Build history of the part. All positions in model axes, mm. Face numbers are marked on the shaded views. Round coordinates to 2 decimals unless told otherwise and drop trailing zeros. Loops run counter-clockwise (first coordinate to the right, second up) from the corner with the lowest first, then second, coordinate; pieces in that order, holes last. Notation, with made-up numbers: (74, -26.5) - (119, -26.5) arc R35 ccw to (119, 11.5) - close; hole circle Ø9 at (4.5, -9.5). An arc over 180 degrees is marked (long way). Use a Markdown table: item, result.
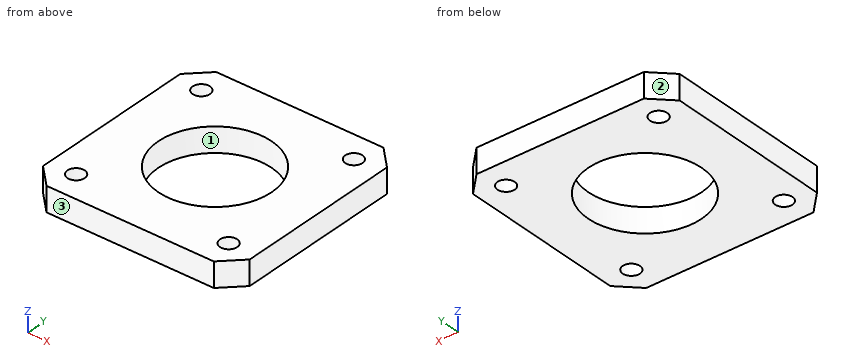
from build123d import *

# Parameters (mm, degrees)
SKETCH_W        = 42
SKETCH_H        = 42
PAD_DEPTH       = 5
SKETCH001_R     = 11.5
POCKET_DEPTH    = 12
SKETCH002_R     = 1.75
POCKET001_DEPTH = 12
CHAMFER_SIZE    = 4


with BuildPart() as part:
    # Sketch → Pad (new body)
    with BuildSketch(Plane.XY):
        Rectangle(SKETCH_W, SKETCH_H)
    extrude(amount=PAD_DEPTH)

    # Sketch001 (on Face6 of Pad) → Pocket (cut)
    with BuildSketch(Plane.XY.offset(5)):
        Circle(SKETCH001_R)
    extrude(amount=-POCKET_DEPTH, mode=Mode.SUBTRACT)

    # Sketch002 (on Face5 of Pocket) → Pocket001 (cut)
    with BuildSketch(Plane.XY.offset(5)):
        with Locations((15.5, 15.5)):
            Circle(SKETCH002_R)
        with Locations((-15.5, 15.5)):
            Circle(SKETCH002_R)
        with Locations((-15.5, -15.5)):
            Circle(SKETCH002_R)
        with Locations((15.5, -15.5)):
            Circle(SKETCH002_R)
    extrude(amount=-POCKET001_DEPTH, mode=Mode.SUBTRACT)

    # Chamfer
    chamfer_edges = [part.edges().sort_by_distance(p)[0] for p in [
        (21, 21, 2.5),
        (-21, 21, 2.5),
        (-21, -21, 2.5),
        (21, -21, 2.5),
    ]]
    chamfer(chamfer_edges, length=CHAMFER_SIZE)


solid = part.part
Q1. Probe line 1 (Y direction, x = -15.5, z = 1.2); line 2 (X direction, y = -16.5, z = 2.15); line 3 (X direction, y = -1.5, z = 1.1). List the from-to ranges inside material, lowest first.
Results found:
| item | result |
|---|---|
| line 1 | y = -21 to -17.25, -13.75 to 13.75, 17.25 to 21 |
| line 2 | x = -21 to -16.94, -14.06 to 14.06, 16.94 to 21 |
| line 3 | x = -21 to -11.4, 11.4 to 21 |
Q2. Cut at C-C, the plane z = 3.35. List the corners of the cut face in (x, y).
Results found:
| item | result |
|---|---|
| outline | (-21, -17) - (-17, -21) - (17, -21) - (21, -17) - (21, 17) - (17, 21) - (-17, 21) - (-21, 17) - close; hole circle Ø3.5 at (-15.5, -15.5); hole circle Ø3.5 at (-15.5, 15.5); hole circle Ø23 at (0, 0); hole circle Ø3.5 at (15.5, -15.5); hole circle Ø3.5 at (15.5, 15.5) |
Q3. Cut at A-A, the plane y = 0. List the corners of the cut face in (x, z).
Results found:
| item | result |
|---|---|
| outline | (-21, 0) - (-11.5, 0) - (-11.5, 5) - (-21, 5) - close; (11.5, 0) - (21, 0) - (21, 5) - (11.5, 5) - close |
Q4. Pull direction Y, two halves, no side cores. Call the marked faces 1, 2 and 3: pulls with the +Y half, pulls with the -Y half, needs draft (parallel to the pull), parting line crosses it, or undercut.
Results found:
| item | result |
|---|---|
| face 1 | undercut |
| face 2 | pulls with the +Y half |
| face 3 | pulls with the -Y half |
Q5. Cut at B-B, the plane y = -15.5. List the corners of the cut face in (x, z).
Results found:
| item | result |
|---|---|
| outline | (-21, 0) - (-17.25, 0) - (-17.25, 5) - (-21, 5) - close; (-13.75, 0) - (13.75, 0) - (13.75, 5) - (-13.75, 5) - close; (17.25, 0) - (21, 0) - (21, 5) - (17.25, 5) - close |
